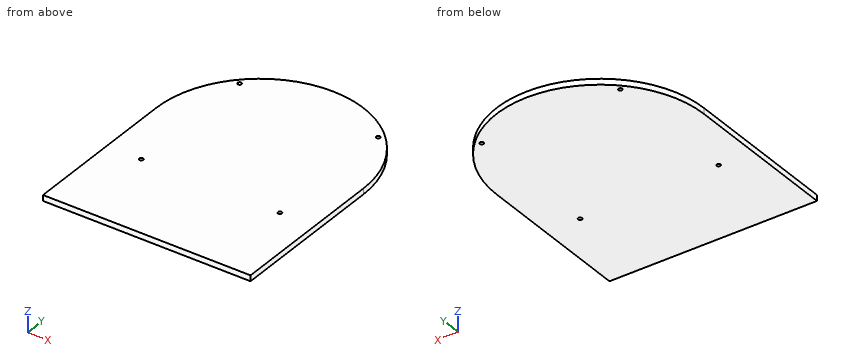
from build123d import *

# Parameters (mm, degrees)
F0_R     = 2.15265
F1_DEPTH = 6.35


with BuildPart() as f1:
    # F0 (on Top) → F1 (new body)
    with BuildSketch(Plane.XY):
        with BuildLine():
            Line((-228.6, -175.571772), (0, -175.571772))
            Line((0, -175.571772), (0, 0))
            ThreePointArc((0, 0), (-114.3, 114.3), (-228.6, 0))
            Line((-228.6, 0), (-228.6, -175.571772))
        make_face()
        with Locations((-190.632177, -76.332177)):
            Circle(F0_R, mode=Mode.SUBTRACT)
        with Locations((-37.967823, -76.332177)):
            Circle(F0_R, mode=Mode.SUBTRACT)
        with Locations((-190.632177, 76.332177)):
            Circle(F0_R, mode=Mode.SUBTRACT)
        with Locations((-37.967823, 76.332177)):
            Circle(F0_R, mode=Mode.SUBTRACT)
    extrude(amount=F1_DEPTH)


solid = f1.part
Input: part model. Units: mm. Frame: model coordinates. Coordinates: 2 decimals unless noted, no trailing zeros. Order: outer loops, then holes, each group sorted by start corner. A loop starts at its lowest first (then second) coordinate and runs counter-clockwise, first axis right, second up. Notation, with made-up numbers: M -31,-5 L 6,-5 A13 cw 6,6 Z; hole C -30.75,2.25 d4. An arc over 180 degrees is marked long. Write item = value, one per line. Start each with the question number.
(1) Line query: line 1 along X through (y, z) = (75, 1.75); line 2 along Y through (x, z) = (-37.5, 2.75); line 3 along Y through (x, z) = (-111.5, 4.5). Output: solid intervals per line, ascending. Write a range as [from, to].
(2) Section A-A on z = 1. Output: boundary loops of the cut face in (x, y), and give its area (3 significant figures).
(3) First-contact query: P1, Ø3.5, axis at x = -190.63, y = 76.33, coming from the +Z side; P2, Ø3, axis at x = -100.5, z = 2, coming from the +Y side. Flat tips, straight axial feed; report the tip coordinate or a pass-through.
(4) Section B-B on x = -62. Output: boundary loops of the cut face in (y, z), and give its area (3 significant figures).
(5) Section C-C on y = 82. Output: boundary loops of the cut face in (x, z), and give its area (3 significant figures).
Result set:
q1.line_1 = [-200.55, -192.32], [-188.94, -39.66], [-36.28, -28.05]
q1.line_2 = [-175.57, -78.43], [-74.23, 74.23], [78.43, 84.65]
q1.line_3 = [-175.57, 114.27]
q2.outline = M -228.6,-175.57 L 0,-175.57 L 0,0 A114.3 ccw -228.6,0 Z; hole C -190.63,-76.33 d4.31; hole C -190.63,76.33 d4.31; hole C -37.97,-76.33 d4.31; hole C -37.97,76.33 d4.31
q2.area = 60,600 mm²
q3.P1 = through
q3.P2 = 113.64
q4.outline = M -175.57,0 L 101.63,0 L 101.63,6.35 L -175.57,6.35 Z
q4.area = 1,760 mm²
q5.outline = M -193.93,0 L -34.67,0 L -34.67,6.35 L -193.93,6.35 Z
q5.area = 1,010 mm²
